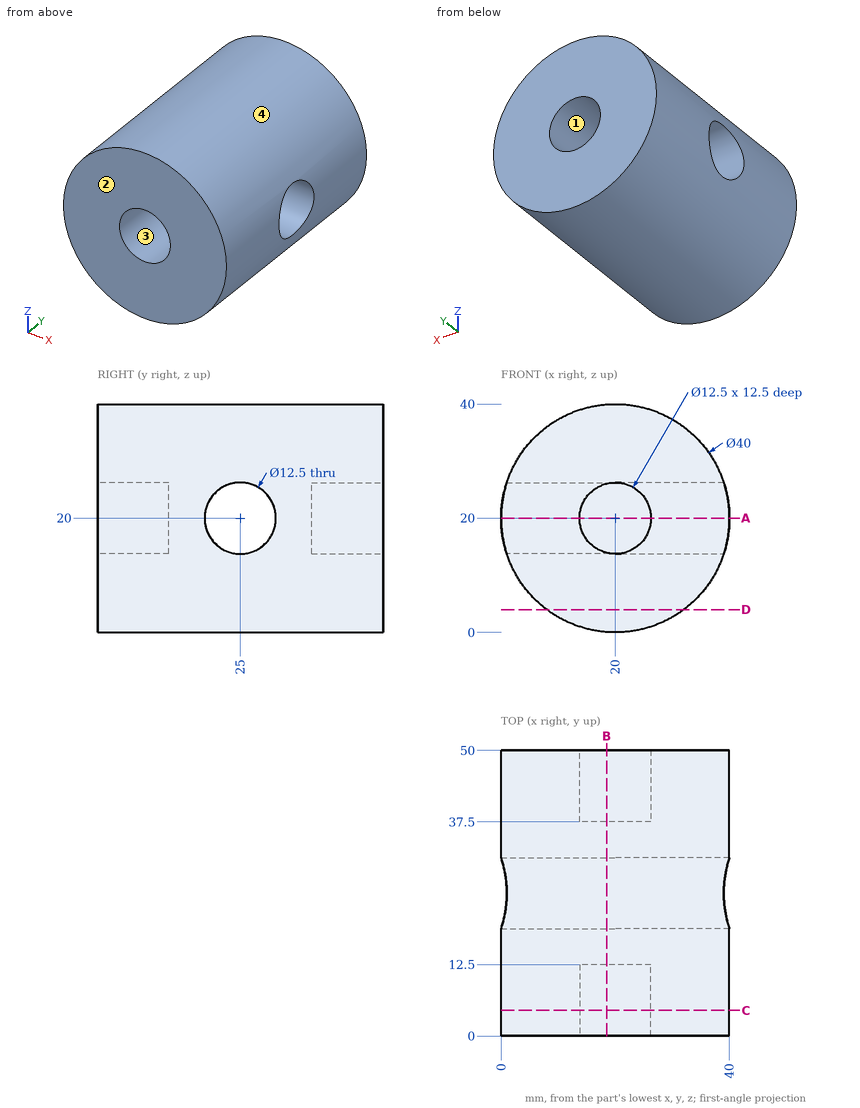
Answer from the drawing. Dimensions are ordinates in mm from the lowest x, y and z of the part. Coordinates: 2 decimals unless noted, no trailing zeros. Loops run counter-clockwise (first coordinate to the right, second up) from the corner with the lowest first, then second, coordinate; pieces in that order, holes last. Notation, with made-up numbers: (-16.5, -29.75) -> (-10.5, -29.75) arc R26 ccw to (-10.5, 7.25) -> close; hole circle Ø1 at (-5.5, 33.25). An arc over 180 degrees is marked (long way). Answer as CSV lines item,"result".
Q1. Each of these flat-tipped pins is pushed along its axis until it touches: pin 1 (10 mm diameter, centred on x = 18, z = 18.5, fed in from -Y); pin 2 (8 mm diameter, centred on y = 28, z = 34, fed in from -X); pin 3 (3 mm diameter, centred on y = 34, z = 7, fed in from -X); pin 4 (10 mm diameter, centred on y = 37.5, z = 4, fed in from -X). Where does it stop, or does it pass through?
Findings:
pin 1,"stops at y = 0"
pin 2,"stops at x = 2.68"
pin 3,"stops at x = 3.64"
pin 4,"stops at x = 3.3"
Q2. Find the intervals of material crossed by probe 1 along Z at (x, y) = (20, 4.25); probe 2 along Z at (x, y) = (22, 5.5); probe 3 along X at (y, z) = (3, 17), in increasing order.
Findings:
probe 1,"z = 0 to 13.75, 26.25 to 40"
probe 2,"z = 0.1 to 14.08, 25.92 to 39.9"
probe 3,"x = 0.23 to 14.52, 25.48 to 39.77"
Q3. The part is cut by section C-C on y = 4.5. Write down the section's boundary in (x, z).
Findings:
outline,"circle Ø40 at (20, 20); hole circle Ø12.5 at (20, 20)"
Q4. The part is cut by section D-D on z = 4. Write down the section's boundary in (x, y), and give its area (3 significant figures).
Findings:
outline,"(8, 0) -> (32, 0) -> (32, 50) -> (8, 50) -> close"
area,"1,200 mm²"
Q5. The part is cut by section B-B on x = 18.5. Write down the section's boundary in (y, z).
Findings:
outline,"(0, 0.06) -> (50, 0.06) -> (50, 13.93) -> (37.5, 13.93) -> (37.5, 26.07) -> (50, 26.07) -> (50, 39.94) -> (0, 39.94) -> (0, 26.07) -> (12.5, 26.07) -> (12.5, 13.93) -> (0, 13.93) -> close; hole circle Ø12.5 at (25, 20)"
Q6. For a pull along Z with two mould halves and no side action, classify the marked faces 1, 2, 3 and 4 as +Z half, -Z half, draft (parallel to the pull), parting line (faces both ways), or undercut.
Findings:
face 1,"undercut"
face 2,"draft"
face 3,"undercut"
face 4,"parting line"
Q7. The part is cut by section A-A on z = 20. Write down the section's boundary in (x, y).
Findings:
outline,"(0, 0) -> (13.75, 0) -> (13.75, 12.5) -> (26.25, 12.5) -> (26.25, 0) -> (40, 0) -> (40, 18.75) -> (0, 18.75) -> close; (0, 31.25) -> (40, 31.25) -> (40, 50) -> (26.25, 50) -> (26.25, 37.5) -> (13.75, 37.5) -> (13.75, 50) -> (0, 50) -> close"
